Geometry check sheet. Reference: the model listing, model coordinates, mm. Face numbers are marked on the shaded views. Give positions to 0.01 mm unless a question says otherwise; leave off trailing zeros. Loops run counter-clockwise (first coordinate to the right, second up) from the corner with the lowest first, then second, coordinate; pieces in that order, holes last.
1. Cross-section at A-A, the plane x = 3.5. Record the cut outline in (y, z), plus the area to 3 significant figures.
2. Material ranges on L1, parallel to X at y = 28.5, z = 36; L2, parallel to Y at x = 1, z = 24; L3, parallel to Y at x = 10.25, z = 46, recorded low to high.
3. Release check for a two-part mould opening along Y. For the marked faces 1, 2 and 3 record: +Y half, -Y half, draft (parallel to the pull), parting line (faces both ways), or undercut.
4. Cross-section at B-B, the plane z = 32. Record the cut outline in (x, y), plus the area to 3 significant figures.
5. Go/stop test with flat-tipped pins: pin 1 Ø1.5 at (y, z) = (28, 41.5) entering from +X; pin 2 Ø1.5 at (x, z) = (9, 23) entering from -Y. Record where each tip stops, or that it passes through.
6. Cross-section at D-D, the plane y = -2. Record the cut outline in (x, z).
7. Cross-section at C-C, the plane x = -2.75. Record the cut outline in (y, z).
from build123d import *

# Parameters (mm, degrees)
SALIENTE_EXTRUIR1_DEPTH = 50
CORTAR_EXTRUIR3_DEPTH   = 5


with BuildPart() as part:
    # Croquis1 → Saliente-Extruir1 (new body)
    with BuildSketch(Plane.XY):
        with BuildLine():
            Line((-5, 31.75), (-5, -31.75))
            Line((-5, -31.75), (9.142135624, -45.892135624))
            ThreePointArc((9.142135624, -45.892135624), (11.642135624, -45.892135624), (11.642135624, -43.392135624))
            Line((11.642135624, -43.392135624), (0, -31.75))
            Line((0, -31.75), (0, 31.75))
            Line((0, 31.75), (11.642135624, 43.392135624))
            ThreePointArc((11.642135624, 43.392135624), (11.642135624, 45.892135624), (9.142135624, 45.892135624))
            Line((9.142135624, 45.892135624), (-5, 31.75))
        make_face()
    extrude(amount=SALIENTE_EXTRUIR1_DEPTH)

    # Croquis4 → Cortar-Extruir3 (cut)
    with BuildSketch(Plane(origin=(0, 0, 0), x_dir=(-1, 0, 0), z_dir=(0, 0, -1))):
        with BuildLine():
            Line((5, 31.75), (-9.142135624, 45.892135624))
            ThreePointArc((-9.142135624, 45.892135624), (-11.642135624, 45.892135624), (-11.642135624, 43.392135624))
            Line((-11.642135624, 43.392135624), (0, 31.75))
            Line((0, 31.75), (0, -31.75))
            Line((0, -31.75), (-11.642135624, -43.392135624))
            ThreePointArc((-11.642135624, -43.392135624), (-11.642135624, -45.892135624), (-9.142135624, -45.892135624))
            Line((-9.142135624, -45.892135624), (5, -31.75))
            Line((5, -31.75), (5, 31.75))
        make_face()
    extrude(amount=-CORTAR_EXTRUIR3_DEPTH, mode=Mode.SUBTRACT)


solid = part.part
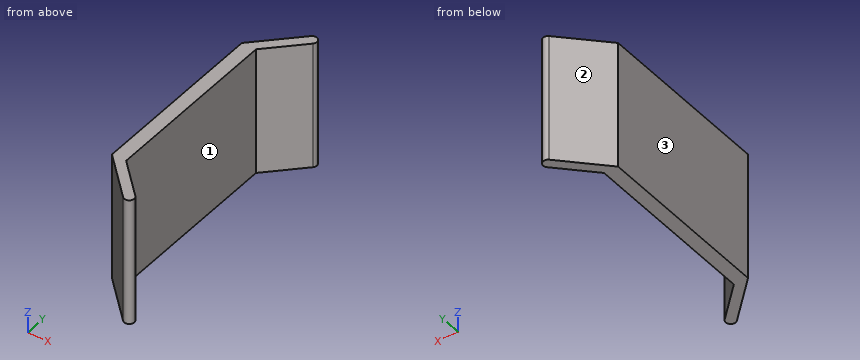
Result:
1. outline: (-40.25, 5) - (-35.25, 5) - (-35.25, 50) - (-40.25, 50) - close; (35.25, 5) - (40.25, 5) - (40.25, 50) - (35.25, 50) - close
1. area: 450 mm2
2. L1: x = -5 to 0
2. L2: y = -37.75 to -32.75, 32.75 to 37.75
2. L3: y = -46.4 to -42, 42 to 46.4
3. face 1: undercut
3. face 2: +Y half
3. face 3: draft
4. outline: (-5, -31.75) - (9.14, -45.89) arc R1.77 ccw to (11.64, -43.39) - (0, -31.75) - (0, 31.75) - (11.64, 43.39) arc R1.77 ccw to (9.14, 45.89) - (-5, 31.75) - close
4. area: 456 mm2
5. pin 1: stops at x = 0
5. pin 2: stops at y = -46.29
6. outline: (-5, 5) - (0, 5) - (0, 50) - (-5, 50) - close
7. outline: (-34, 5) - (34, 5) - (34, 50) - (-34, 50) - close
